from build123d import *

# Parameters (mm, degrees)
CUT_EXTRUDE1_START = 2.3876
CUT_EXTRUDE1_DEPTH = 14.3002
CIRPATTERN1_COUNT  = 10
SKETCH4_R          = 2.38125
CUT_EXTRUDE2_DEPTH = 30.51572079
CUT_EXTRUDE3_DEPTH = 1.7859375


with BuildPart() as part:
    # Sketch2 → Revolve1 (revolve)
    with BuildSketch(Plane(origin=(0, 0, 0), x_dir=(0, 0, -1), z_dir=(1, 0, 0)), mode=Mode.PRIVATE) as revolve1_sk:
        with BuildLine():
            Line((-14.2875, 4.7625), (14.2875, 4.7625))
            Line((14.2875, 4.7625), (14.2875, 18.2626))
            Line((14.2875, 18.2626), (13.10005, 18.2626))
            ThreePointArc((13.10005, 18.2626), (12.234576959, 17.500999922), (11.9126, 16.394017943))
            Line((11.9126, 16.394017943), (11.9126, 14.525435887))
            Line((11.9126, 14.525435887), (-2.3876, 14.525435887))
            Line((-2.3876, 14.525435887), (-2.3876, 16.394017943))
            ThreePointArc((-2.3876, 16.394017943), (-2.709576959, 17.500999922), (-3.57505, 18.2626))
            Line((-3.57505, 18.2626), (-4.7625, 18.2626))
            Line((-4.7625, 18.2626), (-4.7625, 10.3251))
            Line((-4.7625, 10.3251), (-14.2875, 10.3251))
            Line((-14.2875, 10.3251), (-14.2875, 4.7625))
        make_face()
    revolve(revolve1_sk.sketch.rotate(Axis((0, 0, 14.2875), (0, 0, -1)), 90), axis=Axis((0, 0, 14.2875), (0, 0, -1)))

    # Sketch3 → Cut-Extrude1 (cut)
    with BuildSketch(Plane.XY.offset(CUT_EXTRUDE1_START)):
        with BuildLine():
            Line((-1.630736704, 12.4333), (1.630736704, 12.4333))
            Line((1.630736704, 12.4333), (2.3241, 14.3383))
            ThreePointArc((2.3241, 14.3383), (0, 14.525435887), (-2.3241, 14.3383))
            Line((-2.3241, 14.3383), (-1.630736704, 12.4333))
        make_face()
    cut_extrude1 = extrude(amount=-CUT_EXTRUDE1_DEPTH, mode=Mode.SUBTRACT)

    # CirPattern1: Cut-Extrude1 ×10 about axis
    cirpattern1_axis = Axis((0, 0, 0), (0, 0, 1))
    for i in range(1, CIRPATTERN1_COUNT):
        add(cut_extrude1.rotate(cirpattern1_axis, i * 360 / CIRPATTERN1_COUNT), mode=Mode.SUBTRACT)

    # Sketch4 → Cut-Extrude2 (cut, through all)
    with BuildSketch(Plane(origin=(0, 0, 0), x_dir=(0, -1, 0), z_dir=(1, 0, 0))):
        with Locations(Location((0, -9.525, 0), (0, 0, 270))):
            Circle(SKETCH4_R)
    extrude(amount=CUT_EXTRUDE2_DEPTH, mode=Mode.SUBTRACT)

    # Sketch5 → Revolve2 (revolve)
    with BuildSketch(Plane.XY.offset(9.525)):
        Polygon((4.7625, -2.00025), (4.7625, 0), (10.046757609, 0), (10.046757609, -2.00025), (9.665757609, -2.38125), (5.1435, -2.38125), align=None)
    revolve(axis=Axis((4.7625, 0, 9.525), (1, 0, 0)))

    # Sketch6 → Cut-Extrude3 (cut)
    with BuildSketch(Plane(origin=(10.046757609, 5.384140679, 0), x_dir=(0, -1, 0), z_dir=(-1, 0, 0))):
        Polygon((5.384140679, 10.899815329), (4.193515679, 10.212407664), (4.193515679, 8.837592336), (5.384140679, 8.150184671), (6.574765679, 8.837592336), (6.574765679, 10.212407664), align=None)
    extrude(amount=CUT_EXTRUDE3_DEPTH, mode=Mode.SUBTRACT)


solid = part.part
Input: part model. Units: mm. Frame: model coordinates. A direction names the side the tool comes from. Coordinates: 2 decimals unless noted, no trailing zeros. Order: outer loops, then holes, each group sorted by start corner. A loop starts at its lowest first (then second) coordinate and runs counter-clockwise, first axis right, second up. Notation, with made-up numbers: M 3,59.5 L 51,59.5 A8 ccw 51,63.5 Z; hole C 29.25,64.25 d9. An arc over 180 degrees is marked long. Write item = value, one per line. Start each with the question number.
(1) Pull-direction query (Z, two-part tool) for faces 1 (the flat face through (-4, 4, -14.288)), 2 (the flat face through (11.83, -3.82, -4.66)), 3 (the flat face through (8, 8, 4.763)); classes: released by +Z, released by -Z, zero draft, split by the parting line, or undercut.
(2) First-contact query: P1, Ø4.5, axis at y = 0, z = 9.525, coming from the +X side; P2, Ø5, axis at x = 3, z = -7.5, coming from the -Y side; P3, Ø1, axis at x = 1, z = -10, coming from the +Y side. Flat tips, straight axial feed; report the tip coordinate or a pass-through.
(3) Section A-A on x = 0. Output: boundary loops of the cut face in (y, z), and give its area (3 significant figures).
(4) Line query: line 1 along Y through (x, z) = (0, 6.75); line 2 along Y through (x, z) = (-12.5, -10); line 3 along X through (y, z) = (4, 12). Output: solid intervals per line, ascending. Write a range as [from, to].
(5) Reachability of faces 4 (the flat face through (0, 13, 2.388)), 5 (the flat face through (1.982, -13.399, -4.662)), 6 (the cylindrical face through (9.54, 3.95, 9.59)), 7 (the flat face through (9.17, -0.59, 8.49)), 8 (the flat face through (-11.82, -3.86, -4.66)) from +Z, -Z, +X, -X, +Y, -Y: full face, straight path, thin tool, end or side. Return the list, or none.
Result set:
q1.face_1 = released by -Z
q1.face_2 = undercut
q1.face_3 = released by +Z
q2.P1 = 10.05
q2.P2 = -14.34
q2.P3 = 12.43
q3.outline = M -18.26,-14.29 L -4.76,-14.29 L -4.76,14.29 L -10.33,14.29 L -10.33,4.76 L -18.26,4.76 L -18.26,3.58 A2.06 ccw -16.39,2.39 L -12.43,2.39 L -12.43,-11.91 L -16.39,-11.91 A2.06 ccw -18.26,-13.1 Z; M 4.76,-14.29 L 18.26,-14.29 L 18.26,-13.1 A2.06 ccw 16.39,-11.91 L 12.43,-11.91 L 12.43,2.39 L 16.39,2.39 A2.06 ccw 18.26,3.58 L 18.26,4.76 L 10.33,4.76 L 10.33,14.29 L 4.76,14.29 Z
q3.area = 451 mm²
q4.line_1 = [-10.33, -4.76], [4.76, 10.33]
q4.line_2 = [-7.4, -6.31], [-2.29, 2.29], [6.31, 7.4]
q4.line_3 = [-9.52, -2.58], [2.58, 9.52]
q5.face_4 = none
q5.face_5 = -Y
q5.face_6 = +Z
q5.face_7 = +X
q5.face_8 = -X
